Part print with two shaded views. Sizes in mm from the minimum x, y, z corner. A direction names the side the tool comes from. Coordinates: 2 decimals unless noted, no trailing zeros. Order: outer loops, then holes, each group sorted by start corner. A loop starts at its lowest first (then second) coordinate and runs counter-clockwise, first axis right, second up. Notation, with made-up numbers: (48.5, 29) - (61.5, 29) arc R25 cw to (61.5, 68) - close; hole circle Ø7 at (-12.5, 55). An arc over 180 degrees is marked (long way). One line per item, written item: value.
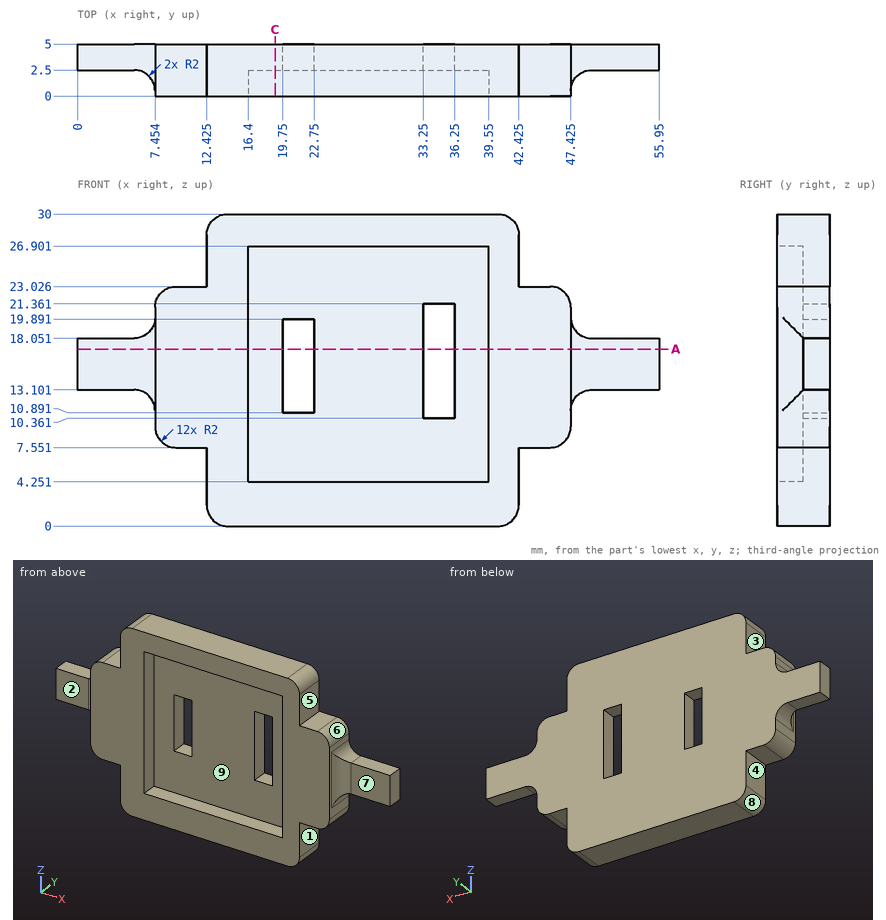
1. Band-saw the part on A-A, the plane z = 17. Count the separate pieces of the cut face and the enclosed holes in it, and give its area (3 significant figures).
Values found:
separate pieces: 3
enclosed holes: 0
area: 169 mm2
2. Band-saw the part on C-C, the plane x = 19. Give the cut face in (y, z).
Values found:
outline: (0, 0) - (5, 0) - (5, 30) - (0, 30) - (0, 26.9) - (2.5, 26.9) - (2.5, 4.25) - (0, 4.25) - close
3. 3-axis set-ups, long thin cutter, end or side, ignore diameter. For the marked faces 1, 2, 3, 4 and 5: which of +Z, -Z, +X, -X, +Y, -Y reach the whole face in a straight line?
Values found:
face 1: -Z, +X, +Y, -Y
face 2: +Z, -Z, -X, -Y
face 3: +Z, -X, +Y, -Y
face 4: -Z, -X, +Y, -Y
face 5: +Z, +X, +Y, -Y
4. Flat gauge pins, fed straight in: P1, Ø2, axis at x = 49.5, y = 3.5, coming from the +Z side; P2, Ø2.5, axis at x = 44.5, y = 3, coming from the +Z side; P3, Ø11.5, axis at x = 23.5, z = 15, coming from the -Y side. Where does each tip first touch, or does it go through?
Values found:
P1: stops at z = 18.28
P2: stops at z = 23.03
P3: stops at y = 2.5
5. Probe line 1 along X through (y, z) = (4.7, 15); line 2 along Z through (x, y) = (37.5, 1); line 3 along Z through (x, y) = (36, 3.5). List the from-to ranges inside material, lowest first.
Values found:
line 1: x = 0 to 19.75, 22.75 to 33.25, 36.25 to 55.95
line 2: z = 0 to 4.25, 26.9 to 30
line 3: z = 0 to 10.36, 21.36 to 30
6. Two-plate mould, pull along Z, no slides. Class the marked faces 6, 7, 8 and 9: pulls with the +Z half, pulls with the -Z half, needs draft (parallel to the pull), parting line crosses it, or undercut.
Values found:
face 6: pulls with the +Z half
face 7: needs draft
face 8: pulls with the -Z half
face 9: undercut
